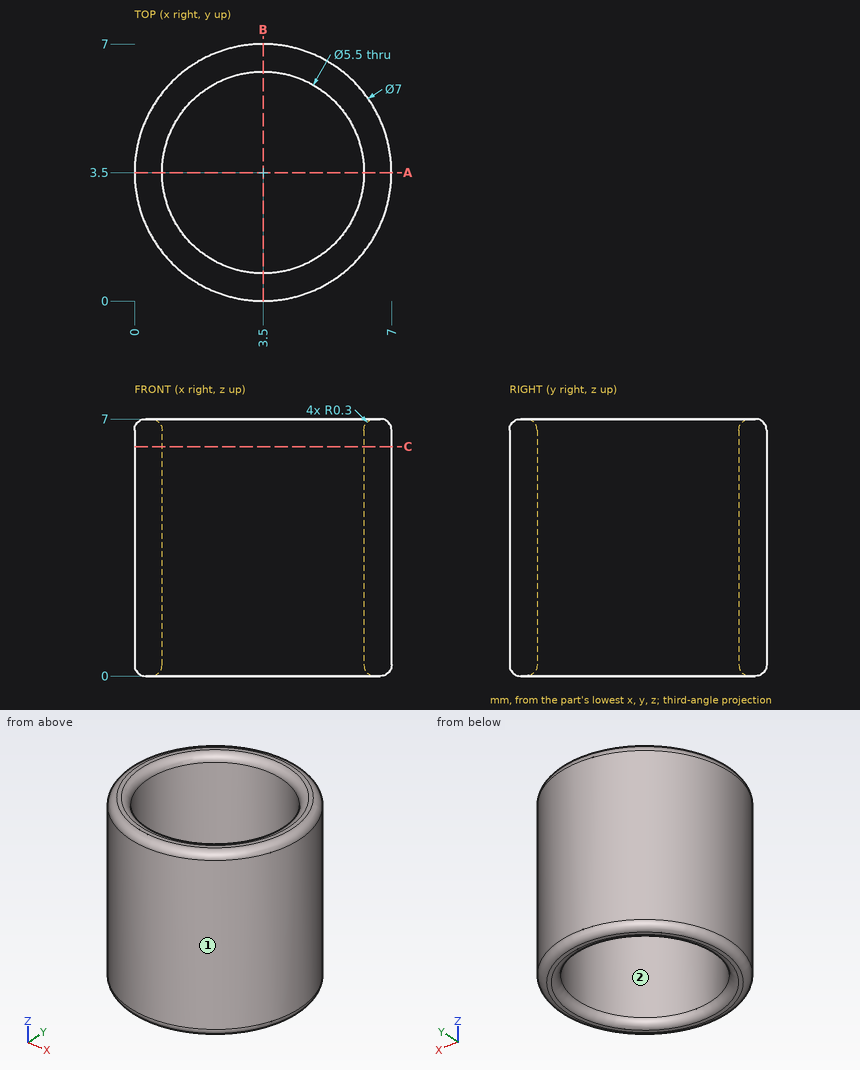
Answer from the drawing. Dimensions are ordinates in mm from the lowest x, y and z of the part. Give positions to 0.01 mm unless a question says otherwise; leave off trailing zeros. Order: outer loops, then holes, each group sorted by start corner. A loop starts at its lowest first (then second) coordinate and runs counter-clockwise, first axis right, second up. Notation, with made-up numbers: (52, 54) -> (66, 54) arc R30 cw to (66, 90) -> close; hole circle Ø9 at (44.5, 36). An arc over 180 degrees is marked (long way). One line per item, written item: value.
Item 1: Find section C-C, the plane z = 6.25. Give the vertices of the cut face in (x, y), plus the area to 3 significant figures.
Answer sheet:
outline: circle Ø7 at (3.5, 3.5); hole circle Ø5.5 at (3.5, 3.5)
area: 14.7 mm²
Item 2: Straight lines are drawn through the part: probe 1 along Y at (x, z) = (3.5, 3.5); probe 2 along X at (y, z) = (1.75, 5); probe 3 along Y at (x, z) = (2.25, 3.75). For each, find the intervals that lie inside material, in ascending order.
Answer sheet:
probe 1: 0 to 0.75, 6.25 to 7
probe 2: 0.47 to 1.38, 5.62 to 6.53
probe 3: 0.23 to 1.05, 5.95 to 6.77
Item 3: Flat-ended cylindrical pins translate along their axes: P1, Ø2, axis at x = 2, z = 1, coming from the +Y side; P2, Ø2, axis at x = 1.5, z = 2, coming from the +Y side; P3, Ø2, axis at x = 1.5, y = 3.5, coming from the -Z side; P4, Ø1.5, axis at x = 3, y = 2, coming from the +Z side. Find the tip coordinate at first contact, or state that the pin passes through.
Answer sheet:
P1: y = 6.96
P2: y = 6.85
P3: z = 0
P4: through
Item 4: Determine the mould class of the marked faces 1 and 2 for opening direction X: released by +X, released by -X, zero draft, split by the parting line, or undercut.
Answer sheet:
face 1: split by the parting line
face 2: undercut
Item 5: Find section A-A, the plane y = 3.5. Give the vertices of the cut face in (x, z).
Answer sheet:
outline: (0, 0.3) arc R0.3 ccw to (0.3, 0) -> (0.45, 0) arc R0.3 ccw to (0.75, 0.3) -> (0.75, 6.7) arc R0.3 ccw to (0.45, 7) -> (0.3, 7) arc R0.3 ccw to (0, 6.7) -> close; (6.25, 0.3) arc R0.3 ccw to (6.55, 0) -> (6.7, 0) arc R0.3 ccw to (7, 0.3) -> (7, 6.7) arc R0.3 ccw to (6.7, 7) -> (6.55, 7) arc R0.3 ccw to (6.25, 6.7) -> close
